Part model, mm, in its own coordinate system. A direction names the side the tool comes from. Give positions to 0.01 mm unless a question says otherwise; leave off trailing zeros. Write each loop counter-clockwise with the first axis right and the second up, starting at its lowest first coordinate (ties: lowest second). Pieces come first, ordered by that corner, then holes. Notation, with made-up numbers: M -34.75,29.25 L 17.25,29.25 A26 ccw 17.25,56.25 Z; hole C 59.25,-13.75 d6. An arc over 180 degrees is marked long. Write item = value, one per line. Start each with the question number.
from build123d import *

# Parameters (mm, degrees)
SKETCH_1_W      = 17
SKETCH_1_H      = 5
SKETCH_1_R      = 1.1
EXTRUDE_1_DEPTH = 2
SKETCH_2_W      = 17
SKETCH_2_H      = 3
EXTRUDE_2_DEPTH = 50
EXTRUDE_3_DEPTH = 12


with BuildPart() as part:
    # 草图1 → 凸台-拉伸1 (new body)
    with BuildSketch(Plane(origin=(0, 0, 0), x_dir=(1, 0, 0), z_dir=(0, 1, 0))):
        Rectangle(SKETCH_1_W, SKETCH_1_H)
        with Locations(Location((5.75, 0, 0), (0, 0, 270))):
            Circle(SKETCH_1_R, mode=Mode.SUBTRACT)
        with Locations(Location((-5.75, 0, 0), (0, 0, 90))):
            Circle(SKETCH_1_R, mode=Mode.SUBTRACT)
        with Locations(Location((0, 0, 0), (0, 0, 270))):
            Circle(SKETCH_1_R, mode=Mode.SUBTRACT)
    extrude(amount=EXTRUDE_1_DEPTH)

    # 草图2 → 凸台-拉伸2 (add)
    with BuildSketch(Plane(origin=(0, 0, 0), x_dir=(1, 0, 0), z_dir=(0, 1, 0))):
        with Locations((0, -4)):
            Rectangle(SKETCH_2_W, SKETCH_2_H)
    extrude(amount=EXTRUDE_2_DEPTH)

    # 草图3 → 凸台-拉伸3 (add)
    with BuildSketch(Plane(origin=(8.5, 0, 0), x_dir=(0, 0, -1), z_dir=(1, 0, 0))):
        Polygon((-5.5, 50), (7, 71.650635095), (10, 71.650635095), (-2.5, 50), align=None)
    extrude(amount=-EXTRUDE_3_DEPTH)


solid = part.part
Q1. Slice it at B-B (z = 0). Give the cut face in (x, y), and give its area (3 significant figures).
Q2. Two-plate mould, pull along X, no slides. Class faces 4 (the face through (1.09, 0.99, -0.14)), 5 (the face through (0, 1, -2.5)), 6 (the face through (-3.5, 62, -2)): +X half, -X half, draft (parallel to the pull), parting line (faces both ways), or undercut.
Q3. Tool access for faces 1 (the face through (2.58, 60.98, -3.84)), 2 (the face through (-6, 50, 4)), 3 (the face through (6.68, 0.99, 0.59)): list every direction of +Z, -Z, +X, -X, +Y, -Y with a clear straight run to the whole face (end or side of a thin tool).
Q4. Slice it at C-C (x = -5.75). Give the cut face in (y, z).
Q5. Probe line 1 along X through (y, z) = (0.5, 0); line 2 along Z through (x, y) = (-5.75, 0.5); line 3 along Y through (x, z) = (-4.5, -2). List the from-to ranges inside material, lowest first.
Q6. Slice it at A-A (x = 0). Give the cut face in (y, z).
Q7. Slice it at D-D (y = 15.5). Give the cut face in (x, z), and give its area (3 significant figures).
Q8. Drop flat-ended pins along their axis: P1, Ø1.5, axis at x = -5.5, z = 3.5, coming from the +Y side; P2, Ø6, axis at x = 4.5, y = 63, coming from the -Z side; P3, Ø8, axis at x = 4, y = 24.5, coming from the -Z side. Give the stop position or say it passes through.
Working result:
q1.outline = M -8.5,0 L -6.85,0 L -6.85,2 L -8.5,2 Z; M -4.65,0 L -1.1,0 L -1.1,2 L -4.65,2 Z; M -3.5,54.33 L 8.5,54.33 L 8.5,59.53 L -3.5,59.53 Z; M 1.1,0 L 4.65,0 L 4.65,2 L 1.1,2 Z; M 6.85,0 L 8.5,0 L 8.5,2 L 6.85,2 Z
q1.area = 83.2 mm2
q2.face_4 = undercut
q2.face_5 = draft
q2.face_6 = -X half
q3.face_1 = -Z, +X, -X
q3.face_2 = +Z, -Z, -X, +Y
q3.face_3 = -Y
q4.outline = M 0,-2.5 L 2,-2.5 L 2,-1.1 L 0,-1.1 Z; M 0,1.1 L 2,1.1 L 2,2.5 L 50,2.5 L 50,5.5 L 0,5.5 Z
q5.line_1 = -8.5 to -6.85, -4.65 to -1.1, 1.1 to 4.65, 6.85 to 8.5
q5.line_2 = -2.5 to -1.1, 1.1 to 5.5
q5.line_3 = 0 to 2
q6.outline = M 0,-2.5 L 2,-2.5 L 2,-1.1 L 0,-1.1 Z; M 0,1.1 L 2,1.1 L 2,2.5 L 50,2.5 L 71.65,-10 L 71.65,-7 L 50,5.5 L 0,5.5 Z
q7.outline = M -8.5,2.5 L 8.5,2.5 L 8.5,5.5 L -8.5,5.5 Z
q7.area = 51.0 mm2
q8.P1 = 50
q8.P2 = -6.74
q8.P3 = 2.5
